```python
from build123d import *

# Parameters (mm, degrees)
BOSS_EXTRUDE1_DEPTH      = 33.5
SKETCH2_W                = 20
SKETCH2_H                = 2.5
BOSS_EXTRUDE2_DEPTH      = 8
CUT_EXTRUDE5_DEPTH       = 12
RESSALTO_EXTRUS_O4_DEPTH = 0.75
SKETCH6_R                = 1.5
CUT_EXTRUDE6_DEPTH       = 12
CUT_EXTRUDE8_REACH       = 49.447
SKETCH14_W               = 1.6
SKETCH14_H               = 5
SKETCH9_R                = 1
CORTE_EXTRUS_O1_DEPTH    = 54.324478432
FILETE1_R                = 3
ESBO_O6_R                = 1
CORTE_EXTRUS_O6_DEPTH    = 2
ESBO_O8_W                = 0.75
ESBO_O8_H                = 19
ESBO_O8_H_2              = 14
CORTE_EXTRUS_O8_DEPTH    = 48.44733923
FILETE1_OF_ESPELHAR1_R   = 3
CORTE_EXTRUS_O9_DEPTH    = 48.44733923
CORTE_EXTRUS_O10_DEPTH   = 61.891809882


with BuildPart() as part:
    # Sketch1 → Boss-Extrude1 (new body)
    with BuildSketch(Plane.XY):
        Polygon((17, -20), (19, -20), (19, 14), (-19, 14), (-19, -20), (-17, -20), (-17, -1), (17, -1), align=None)
    extrude(amount=BOSS_EXTRUDE1_DEPTH)

    # Sketch2 → Boss-Extrude2 (add)
    with BuildSketch(Plane(origin=(19, 0, 0), x_dir=(0, 0, -1), z_dir=(1, 0, 0))):
        with Locations((-23.5, -18.75)):
            Rectangle(SKETCH2_W, SKETCH2_H)
    boss_extrude2 = extrude(amount=BOSS_EXTRUDE2_DEPTH)

    # Sketch12 → Cut-Extrude5 (cut)
    with BuildSketch(Plane(origin=(0, 14, 0), x_dir=(1, 0, 0), z_dir=(0, 1, 0))):
        Polygon((-7.535857559, -4.75), (-7.535857559, -28.75), (-3.035857559, -28.75), (-3.035857559, -33.5), (1.964142441, -33.5), (1.964142441, -28.75), (12.664142441, -28.75), (12.664142441, -33.5), (19, -33.5), (19, 0), (12.664142441, 0), (12.664142441, -4.75), align=None)
    extrude(amount=-CUT_EXTRUDE5_DEPTH, mode=Mode.SUBTRACT)

    # Esboço10 → Ressalto-extrusão4 (add)
    with BuildSketch(Plane(origin=(19, 0, 0), x_dir=(0, 0, -1), z_dir=(1, 0, 0))):
        Polygon((-33.5, 2), (0, 2), (0, -17.5), (0, -20), (-13.5, -20), (-13.5, -17.5), (-33.5, -17.5), align=None)
    ressalto_extrus_o4 = extrude(amount=RESSALTO_EXTRUS_O4_DEPTH)

    # Sketch6 → Cut-Extrude6 (cut)
    with BuildSketch(Plane(origin=(12.664142441, 0, 0), x_dir=(0, 0, -1), z_dir=(1, 0, 0))):
        with Locations((-31.125, 8)):
            Circle(SKETCH6_R)
    cut_extrude6 = extrude(amount=-CUT_EXTRUDE6_DEPTH, mode=Mode.SUBTRACT)

    # Sketch14 → Cut-Extrude8 (cut, up to next)
    with BuildSketch(Plane.XY.offset(33.5), mode=Mode.PRIVATE) as cut_extrude8_sk1:
        with Locations((6.664142441, 8)):
            Rectangle(SKETCH14_W, SKETCH14_H)
    cut_extrude8_tool1 = extrude(cut_extrude8_sk1.sketch, amount=-CUT_EXTRUDE8_REACH, mode=Mode.PRIVATE) & part.part
    cut_extrude8 = cut_extrude8_tool1.solids().sort_by_distance((6.664142, 8, 33.5))[0]
    add(cut_extrude8, mode=Mode.SUBTRACT)

    # Mirror6: Cut-Extrude6, Cut-Extrude8 across plane
    add(cut_extrude6.mirror(Plane.XY.offset(16.75)), mode=Mode.SUBTRACT)
    add(cut_extrude8.mirror(Plane.XY.offset(16.75)), mode=Mode.SUBTRACT)

    # Sketch9 → Corte-extrusão1 (cut, through all)
    with BuildSketch(Plane(origin=(0, -17.5, 0), x_dir=(1, 0, 0), z_dir=(0, 1, 0))):
        with Locations(Location((23, -16.5, 0), (0, 0, 270))):
            Circle(SKETCH9_R)
        with Locations(Location((23, -30.5, 0), (0, 0, 270))):
            Circle(SKETCH9_R)
    corte_extrus_o1 = extrude(amount=-CORTE_EXTRUS_O1_DEPTH, mode=Mode.SUBTRACT)

    # Filete1
    filete1_edges = [part.edges().sort_by_distance(p)[0] for p in [
        (27, -18.75, 13.5),
        (27, -18.75, 33.5),
    ]]
    fillet(filete1_edges, radius=FILETE1_R)

    # Esboço6 → Corte-extrusão6 (cut)
    with BuildSketch(Plane.ZY.offset(19)):
        with Locations((22.25, 8)):
            Circle(ESBO_O6_R)
    extrude(amount=-CORTE_EXTRUS_O6_DEPTH, mode=Mode.SUBTRACT)

    # Esboço8 → Corte-extrusão8 (cut, through all)
    with BuildSketch(Plane.XY.offset(33.5)):
        with Locations((17.375, -10.5)):
            Rectangle(ESBO_O8_W, ESBO_O8_H)
        with Locations((-17.375, -8)):
            Rectangle(ESBO_O8_W, ESBO_O8_H_2)
    corte_extrus_o8 = extrude(amount=-CORTE_EXTRUS_O8_DEPTH, mode=Mode.SUBTRACT)

    # Espelhar1: Boss-Extrude2, Ressalto-extrusão4, Corte-extrusão1, Corte-extrusão8 across plane
    add(boss_extrude2.mirror(Plane(origin=(0, 0, 0), x_dir=(0, 0, 1), z_dir=(1, 0, 0))))
    add(ressalto_extrus_o4.mirror(Plane(origin=(0, 0, 0), x_dir=(0, 0, 1), z_dir=(1, 0, 0))))
    add(corte_extrus_o1.mirror(Plane(origin=(0, 0, 0), x_dir=(0, 0, 1), z_dir=(1, 0, 0))), mode=Mode.SUBTRACT)
    add(corte_extrus_o8.mirror(Plane(origin=(0, 0, 0), x_dir=(0, 0, 1), z_dir=(1, 0, 0))), mode=Mode.SUBTRACT)

    # Filete1 of Espelhar1
    filete1_of_espelhar1_edges = [part.edges().sort_by_distance(p)[0] for p in [
        (-27, -18.75, 13.5),
        (-27, -18.75, 33.5),
    ]]
    fillet(filete1_of_espelhar1_edges, radius=FILETE1_OF_ESPELHAR1_R)

    # Esboço11 → Corte-extrusão9 (cut, through all)
    with BuildSketch(Plane.XY.offset(33.5)):
        with BuildLine():
            Line((-17.75, -1), (17.75, -1))
            add(Edge.make_bspline(
                [(-17.75, -1), (0, 1.838465609), (17.75, -1)],
                knots=[0, 0, 0, 1, 1, 1], degree=2))
        make_face()
    extrude(amount=-CORTE_EXTRUS_O9_DEPTH, mode=Mode.SUBTRACT)

    # Esboço12 → Corte-extrusão10 (cut, through all)
    with BuildSketch(Plane(origin=(19.75, 0, 0), x_dir=(0, 0, -1), z_dir=(1, 0, 0))):
        with BuildLine():
            Line((0, -20), (-13.5, -20))
            Line((-13.5, -20), (-13.5, -12))
            ThreePointArc((-13.5, -12), (-11.742640687, -7.757359313), (-7.5, -6))
            Line((-7.5, -6), (0, -6))
            Line((0, -6), (0, -20))
        make_face()
    extrude(amount=-CORTE_EXTRUS_O10_DEPTH, mode=Mode.SUBTRACT)


solid = part.part
```
Read the model definition and answer for the solid it produces. Units are mm, in the model's axes. A direction names the side the tool comes from. Coordinates: 2 decimals unless noted, no trailing zeros. Order: outer loops, then holes, each group sorted by start corner. A loop starts at its lowest first (then second) coordinate and runs counter-clockwise, first axis right, second up. Notation, with made-up numbers: (22, -21.75) - (56, -21.75) arc R35 ccw to (56, 14.25) - close; hole circle Ø1 at (-5.5, -11.75). An arc over 180 degrees is marked (long way). Answer as a JSON object with one key per item and string values. Group by question number.
Item 1: Flat-ended cylindrical pins translate along their axes: P1, Ø3, axis at x = 19.5, y = -15, coming from the -Z side; P2, Ø1.5, axis at y = -5, z = 19.5, coming from the +X side; P3, Ø2.5, axis at x = -23, z = 30.5, coming from the +Y side. Find the tip coordinate at first contact, or state that the pin passes through.
Item 2: Section D-D (y = 1) is taken. Give the vertices of the cut face in (x, z), plus the area to 3 significant figures.
Item 3: Section C-C (y = 8) is taken. State how many separate pieces and enclosed holes the cut face has, plus the area to 4 significant figures.
Item 4: The mould has two halves that part along Z. Classify faces 5 (the face through (26.1, -18.73, 32.64)), 6 (the face through (22.11, -18.73, 16.96)), 7 (the face through (7, 10.5, 31)): +Z half, -Z half, draft (parallel to the pull), parting line (faces both ways), or undercut.
Item 5: Section B-B (y = -14) is taken. Give the vertices of the cut face in (x, z), plus the area to 3 significant figures.
Item 6: Consider probe 1 along X at (y, z) = (-19.05, 16.5); probe 2 along X at (y, z) = (9.5, 32.5); probe 3 along X at (y, z) = (-17, 21). Determine where each line is inside the solid, lowest interval first. Write a range as from..to.
Item 7: Section A-A (x = -23) is taken. Give the vertices of the cut face in (y, z), plus the area to 3 significant figures.
Item 8: A tool of negligible diameter and unlimited length cuts with its end or side. For faces 1 (the face through (-17.75, -9, 21)), 2 (the face through (-19, -6, 4)), 3 (the face through (19.75, -5, 20)), 4 (the face through (-19, 8, 17)), from which of +Z, -Z, +X, -X, +Y, -Y can it reach the whole face along a straight path? Write none if from no direction.
Results are:
{
 "1": {"P1": "stops at z = 13.5", "P2": "stops at x = 19.75", "P3": "stops at y = -17.5"},
 "2": {"outline": "(-19.75, 0) - (19.75, 0) - (19.75, 33.5) - (-19.75, 33.5) - close", "area": "1,320 mm^2"},
 "3": {"separate pieces": "7", "enclosed holes": "0", "area": "474.5 mm^2"},
 "4": {"face 5": "+Z half", "face 6": "undercut", "face 7": "draft"},
 "5": {"outline": "(-19.75, 13.5) - (-17.75, 13.5) - (-17.75, 33.5) - (-19.75, 33.5) - close; (17.75, 13.5) - (19.75, 13.5) - (19.75, 33.5) - (17.75, 33.5) - close", "area": "80.0 mm^2"},
 "6": {"probe 1": "x = -27..-24, -22..-17.75, 17.75..22, 24..27", "probe 2": "x = -19..-3.04, 1.96..5.86, 7.46..12.66", "probe 3": "x = -19.75..-17.75, 17.75..19.75"},
 "7": {"outline": "(-20, 13.5) - (-17.5, 13.5) - (-17.5, 15.5) - (-20, 15.5) - close; (-20, 17.5) - (-17.5, 17.5) - (-17.5, 29.5) - (-20, 29.5) - close; (-20, 31.5) - (-17.5, 31.5) - (-17.5, 33.5) - (-20, 33.5) - close", "area": "40.0 mm^2"},
 "8": {"face 1": "+Z, -Z, -Y", "face 2": "-Z, +X, -X, -Y", "face 3": "+Z, -Z, +X, +Y", "face 4": "+Z, -Z, -X, +Y"}
}
